Autodesk Inventor part; units mm, degrees
ref_plane "YZ Plane" through (0, 0, 0) normal (1, 0, 0) x (0, 1, 0)
ref_plane "XZ Plane" through (0, 0, 0) normal (0, 1, 0) x (-1, 0, 0)
ref_plane "XY Plane" through (0, 0, 0) normal (0, 0, 1) x (1, 0, 0)
sketch "Sketch1" plane through (0, 0, 0) normal (0, 0, 1) x (1, 0, 0)
  circle A0 centre (0, 132.2876) radius 225 construction
  circle A1 centre (0, 132.2876) radius 200 construction
  line L0 (150, 132.2876) -> (150, 0) construction
  line L1 (150, 0) -> (0, 0)
  line L2 (0, 0) -> (0, -92.7124)
  arc A2 (0, -92.7124) -> (175, -9.1338) centre (0, 132.2876) ccw
  line L3 (157.5, 0) -> (157.5, 10)
  line L4 (157.5, 10) -> (167.5, 10)
  line L5 (167.5, 10) -> (167.5, 0)
  line L6 (150, 0) -> (157.5, 0)
  line L7 (175, -35.9935) -> (175, -9.1338) construction
  line L8 (175, 0) -> (175, -9.1338)
  line L9 (167.5, 0) -> (175, 0)
  line L10 (0, 132.2876) -> (0, -92.7124) construction
  line L11 (0, 132.2876) -> (225, 132.2876) construction
  line L12 (0, 0) -> (130.6185, 0) construction
  dimension "d0" = 450
  dimension "d1" = 25
  dimension "d3" = 10
  dimension "d4" = 10
  dimension "d6" = 7.5
  dimension "d7" = 90
  dimension "d9" = 25
  dimension "d12" = 90
  dimension "d13" = 75
  dimension "d14" = 90
extrude "Extrusion1" add sketch "Sketch1" along normal blind 15
sketch "Sketch2" plane through (0, 0, 15) normal (0, 0, 1) x (1, 0, 0)
  line L0 (0, 0) -> (0, -92.7124)
  line L1 (0, -15) -> (10, -15)
  line L2 (10, -15) -> (10, -25)
  line L3 (10, -25) -> (0, -25)
  line L4 (0, -25) -> (0, -15)
  line L5 (0, -50) -> (10, -50)
  line L6 (10, -50) -> (10, -60)
  line L7 (10, -60) -> (0, -60)
  line L8 (0, -60) -> (0, -50)
  line L9 (157.5, 0) -> (0, 0)
  dimension "d15" = 10
  dimension "d16" = 10
  dimension "d17" = 10
  dimension "d18" = 10
  dimension "d19" = 25
  dimension "d20" = 15
extrude "Extrusion2" cut sketch "Sketch2" against normal blind 15
sketch "Sketch3" plane through (0, 0, 15) normal (0, 0, 1) x (1, 0, 0)
  line L0 (157.5, 0) -> (0, 0) construction
  line L1 (25, 0) -> (125, 0) construction
  line L2 (125, 0) -> (125, -20) construction
  line L3 (125, -20) -> (25, -20) construction
  line L4 (25, -20) -> (25, 0) construction
  circle A0 centre (50, -10) radius 2.5
  circle A1 centre (100, -10) radius 2.5
  dimension "d23" = 100
  dimension "d24" = 20
  dimension "d25" = 25
  dimension "d26" = 5
  dimension "d27" = 5
  dimension "d28" = 25
  dimension "d29" = 25
extrude "Extrusion3" cut sketch "Sketch3" against normal through all
thread "Thread1"
thread "Thread2"
sketch "Sketch4" plane through (0, 0, 15) normal (0, 0, 1) x (1, 0, 0)
  line L0 (157.5, 0) -> (0, 0)
  line L1 (25, 0) -> (125, 0)
  line L2 (125, 0) -> (125, -20)
  line L3 (125, -20) -> (25, -20)
  line L4 (25, -20) -> (25, 0)
  dimension "d36" = 100
  dimension "d37" = 20
  dimension "d38" = 25
extrude "Extrusion4" cut sketch "Sketch4" against normal blind 5
sketch "Sketch5" plane through (0, 0, 15) normal (0, 0, 1) x (1, 0, 0)
  circle A0 centre (0, 132.2876) radius 225 construction
  arc A1 (0, -92.7124) -> (175, -9.1338) centre (0, 132.2876) ccw construction
  circle A2 centre (0, 132.2876) radius 210 construction
  circle A3 centre (144.4906, -20.1016) radius 2.5
  circle A4 centre (155, -9.3987) radius 2.5
  line L0 (175, -9.1338) -> (175, 0)
  point P0 (0, 0)
  dimension "d41" = 450
  dimension "d42" = 15
  dimension "d43" = 5
  dimension "d44" = 5
  dimension "d45" = 15
  dimension "d46" = 20
extrude "Extrusion5" cut sketch "Sketch5" against normal through all
thread "Thread3"
thread "Thread4"
sketch "Sketch6" plane through (0, 0, 15) normal (0, 0, 1) x (1, 0, 0)
  circle A0 centre (69.0912, -25.1338) radius 2.5
  circle A1 centre (84.0912, -25.1338) radius 2.5
  line L0 (25, 0) -> (125, 0)
  arc A2 (0, -92.7124) -> (175, -9.1338) centre (0, 132.2876) ccw construction
  line L1 (175, -9.1338) -> (-10.7224, -9.1338) construction
  line L2 (0, 0) -> (0, -15) construction
  dimension "d53" = 5
  dimension "d54" = 5
  dimension "d56" = 16
  dimension "d57" = 69.0912
  dimension "d58" = 15
extrude "Extrusion6" cut sketch "Sketch6" against normal through all
thread "Thread5"
thread "Thread6"
properties part number "CP003" material "ABS Plastic"
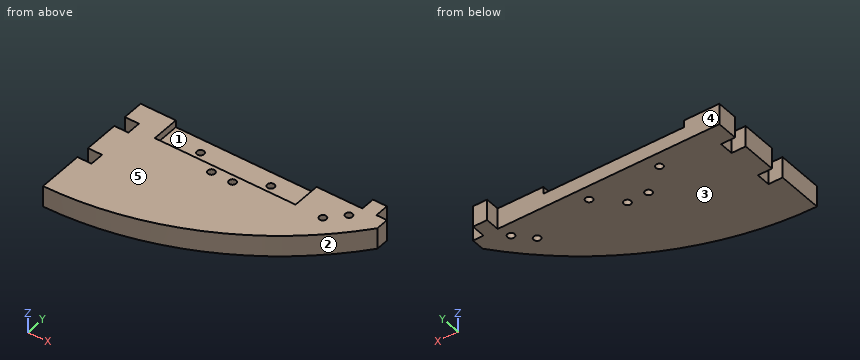
Could you check a few things on this model? Use its own coordinates, in mm. Face numbers are marked on the shaded views. A direction names the side the tool comes from. Give positions to 0.01 mm unless a question says otherwise; leave off trailing zeros. Order: outer loops, then holes, each group sorted by start corner. A loop starts at its lowest first (then second) coordinate and runs counter-clockwise, first axis right, second up.
Item 1: If we mould it in two halves opening along X, with no side actions, what happens to the marked faces 1, 2 and 3? For each: pulls with the +X half, pulls with the -X half, needs draft (parallel to the pull), parting line crosses it, or undercut.
Item 2: If we section it at B-B, the plane x = 50: Write out the boundary of the cut face in (y, z).
Item 3: If we section it at A-A, the plane y = -4: Write out the boundary of the cut face in (x, z).
Item 4: I need wall thicknesses on line 1 (Y direction, x = 100, z = 4.5); line 2 (Z direction, x = 121.5, y = -6); line 3 (Y direction, x = 50, z = 2.25). Which ranges of each line are inside material? Lowest first, please.
Item 5: I'm going to push flat-ended pins straight in: pin 1 (2.5 mm diameter, centred on y = -12, z = 13.5, fed in from +X); pin 2 (2 mm diameter, centred on y = -28, z = 4.5, fed in from +X); pin 3 (3 mm diameter, centred on x = 2.5, z = 9.5, fed in from +Y). Where does each tip first touch, or does it pass through?
Item 6: If we section it at C-C, the plane z = 4: Write out the boundary of the cut face in (x, y), plus the area to 3 significant figures.
Item 7: For the marked faces 4 and 5, which set-ups out of +Z, -Z, +X, -X, +Y, -Y let a thin tool reach every point of the face, with its end or its side?
Item 8: If we section it at D-D, the plane x = 155: Write out the boundary of the cut face in (y, z).
Values:
1. face 1: undercut
1. face 2: pulls with the +X half
1. face 3: needs draft
2. outline: (-87.09, 0) - (-12.5, 0) - (-12.5, 10) - (-20, 10) - (-20, 15) - (-87.09, 15) - close; (-7.5, 0) - (0, 0) - (0, 10) - (-7.5, 10) - close
3. outline: (0, 0) - (175, 0) - (175, 15) - (125, 15) - (125, 10) - (25, 10) - (25, 15) - (0, 15) - close
4. line 1: y = -69.27 to -12.5, -7.5 to 0
4. line 2: z = 0 to 10
4. line 3: y = -87.09 to -12.5, -7.5 to 0
5. pin 1: stops at x = 173.68
5. pin 2: stops at x = 158.91
5. pin 3: stops at y = 0
6. outline: (0, -92.71) arc R225 ccw to (175, -9.13) - (175, 0) - (167.5, 0) - (167.5, 10) - (157.5, 10) - (157.5, 0) - (0, 0) - (0, -15) - (10, -15) - (10, -25) - (0, -25) - (0, -50) - (10, -50) - (10, -60) - (0, -60) - close; hole circle Ø5 at (50, -10); hole circle Ø5 at (69.09, -25.13); hole circle Ø5 at (84.09, -25.13); hole circle Ø5 at (100, -10); hole circle Ø5 at (144.49, -20.1); hole circle Ø5 at (155, -9.4)
6. area: 11,600 mm2
7. face 4: +Z, -Z, -X, +Y
7. face 5: +Z, +X, -X, +Y, -Y
8. outline: (-30.81, 0) - (-11.9, 0) - (-11.9, 15) - (-30.81, 15) - close; (-6.9, 0) - (0, 0) - (0, 15) - (-6.9, 15) - close
